from build123d import *

# Parameters (mm, degrees)
F0_W     = 3.2558272286
F0_H     = 15.3517797806
F1_DEPTH = 20
F2_R     = 2


with BuildPart() as f1:
    # F0 (on Top) → F1 (new body)
    with BuildSketch(Plane.XY):
        with BuildLine():
            Line((-40, -25), (40, -25))
            Line((40, -25), (40, 20))
            ThreePointArc((40, 20), (38.5355339059, 23.5355339059), (35, 25))
            Line((35, 25), (-35, 25))
            ThreePointArc((-35, 25), (-38.5355339059, 23.5355339059), (-40, 20))
            Line((-40, 20), (-40, -25))
        make_face()
        with BuildLine():
            Line((-12.7209101006, -4.8896298527), (-16.6285747722, -20.2414096333))
            Line((-16.6285747722, -20.2414096333), (-20.3346402347, -20.2414096333))
            Line((-20.3346402347, -20.2414096333), (-22.4144720763, -12.1774412653))
            add(Edge.make_bspline(
                [(-22.4144720763, -12.1774412653), (-22.5287116282, -11.7473629523), (-22.8075905342, -10.3983282441)],
                knots=[0, 0, 0, 1, 1, 1], degree=2))
            add(Edge.make_bspline(
                [(-22.8075905342, -10.3983282441), (-23.0864694403, -9.0492935358), (-23.1267892821, -8.5856153547)],
                knots=[0, 0, 0, 1, 1, 1], degree=2))
            add(Edge.make_bspline(
                [(-23.1267892821, -8.5856153547), (-23.1906290317, -9.1534531273), (-23.4426280432, -10.4084082045)],
                knots=[0, 0, 0, 1, 1, 1], degree=2))
            add(Edge.make_bspline(
                [(-23.4426280432, -10.4084082045), (-23.6946270547, -11.6633632818), (-23.8323865143, -12.1976011862)],
                knots=[0, 0, 0, 1, 1, 1], degree=2))
            Line((-23.8323865143, -12.1976011862), (-25.8987784087, -20.2414096333))
            Line((-25.8987784087, -20.2414096333), (-29.5947639107, -20.2414096333))
            Line((-29.5947639107, -20.2414096333), (-33.5125085428, -4.8896298527))
            Line((-33.5125085428, -4.8896298527), (-30.3104411033, -4.8896298527))
            Line((-30.3104411033, -4.8896298527), (-28.3448488136, -13.2694369818))
            add(Edge.make_bspline(
                [(-28.3448488136, -13.2694369818), (-27.8307708302, -15.5911878744), (-27.6022917264, -17.2913412053)],
                knots=[0, 0, 0, 1, 1, 1], degree=2))
            add(Edge.make_bspline(
                [(-27.6022917264, -17.2913412053), (-27.5384519768, -16.6932635514), (-27.3116528665, -15.4383084741)],
                knots=[0, 0, 0, 1, 1, 1], degree=2))
            add(Edge.make_bspline(
                [(-27.3116528665, -15.4383084741), (-27.0848537561, -14.1833533968), (-26.8866145337, -13.4911961119)],
                knots=[0, 0, 0, 1, 1, 1], degree=2))
            Line((-26.8866145337, -13.4911961119), (-24.6488633116, -4.8896298527))
            Line((-24.6488633116, -4.8896298527), (-21.5744753713, -4.8896298527))
            Line((-21.5744753713, -4.8896298527), (-19.3367241492, -13.4911961119))
            add(Edge.make_bspline(
                [(-19.3367241492, -13.4911961119), (-19.1888847291, -14.0657538581), (-18.9688055924, -15.253509199)],
                knots=[0, 0, 0, 1, 1, 1], degree=2))
            add(Edge.make_bspline(
                [(-18.9688055924, -15.253509199), (-18.7487264557, -16.4412645399), (-18.6344869038, -17.2913412053)],
                knots=[0, 0, 0, 1, 1, 1], degree=2))
            add(Edge.make_bspline(
                [(-18.6344869038, -17.2913412053), (-18.5303273124, -16.4715044213), (-18.2984882218, -15.2484692188)],
                knots=[0, 0, 0, 1, 1, 1], degree=2))
            add(Edge.make_bspline(
                [(-18.2984882218, -15.2484692188), (-18.0666491312, -14.0254340163), (-17.8784898693, -13.2694369818)],
                knots=[0, 0, 0, 1, 1, 1], degree=2))
            Line((-17.8784898693, -13.2694369818), (-15.9263375269, -4.8896298527))
            Line((-15.9263375269, -4.8896298527), (-12.7209101006, -4.8896298527))
        make_face(mode=Mode.SUBTRACT)
        with Locations((-9.1610040648, -12.565519743)):
            Rectangle(F0_W, F0_H, mode=Mode.SUBTRACT)
        Polygon((5.8127771986, -20.2414096333), (-3.6691056075, -20.2414096333), (-3.6691056075, -4.8896298527), (-0.4132783789, -4.8896298527), (-0.4132783789, -17.5534201773), (5.8127771986, -17.5534201773), align=None, mode=Mode.SUBTRACT)
        Polygon((17.9624895398, -20.2414096333), (8.4806067337, -20.2414096333), (8.4806067337, -4.8896298527), (11.7364339623, -4.8896298527), (11.7364339623, -17.5534201773), (17.9624895398, -17.5534201773), align=None, mode=Mode.SUBTRACT)
        Polygon((22.2263128144, -4.8896298527), (25.4082203329, -11.2097650611), (28.6102877724, -4.8896298527), (32.1181140125, -4.8896298527), (27.0243739934, -14.2673530673), (27.0243739934, -20.2414096333), (23.7920666725, -20.2414096333), (23.7920666725, -14.3715126587), (18.6983266534, -4.8896298527), align=None, mode=Mode.SUBTRACT)
    extrude(amount=F1_DEPTH)

    # F2
    f2_edges = [f1.edges().sort_by_distance(p)[0] for p in [
        (-40, -2.5, 20),
    ]]
    fillet(f2_edges, radius=F2_R)


solid = f1.part
Source: CAD feature listing. Evaluate the final solid. Frame: model axes, mm. Give positions to 0.01 mm unless a question says otherwise; leave off trailing zeros. Loops run counter-clockwise (first coordinate to the right, second up) from the corner with the lowest first, then second, coordinate; pieces in that order, holes last. Notation, with made-up numbers: (68.25, 40.5) -> (89.25, 40.5) arc R35 cw to (89.25, 75.5) -> close; hole circle Ø1 at (-7, 54.5). An arc over 180 degrees is marked (long way). Use a Markdown table: item, result. Add a question column.
1) Section query B-B, the plane y = -19. Count the separate pieces of the cut face and the enclosed holes in it, then the cut area to 3 significant figures.
2) Section query A-A, the plane x = 15.5. Return the cut outline in (y, z).
3) Line query: line 1 along Y through (x, z) = (3, 4.5); line 2 along Y through (x, z) = (30.5, 8); line 3 along X through (y, z) = (20.5, 6.5). Output: solid intervals per line, ascending. Write a range as [from, to].
4) Pull-direction query (Y, two-part tool) for faces 1 (the face through (-1, 0, 0)), 2 (the face through (25, -20.241, 10)), 3 (the face through (-10.789, -13, 10)); classes: +Y half, -Y half, draft (parallel to the pull), parting line (faces both ways), or undercut.
Numbers:
| question | item | result |
|---|---|---|
| 1 | separate pieces | 7 |
| 1 | enclosed holes | 0 |
| 1 | area | 916 mm2 |
| 2 | outline | (-25, 0) -> (-20.24, 0) -> (-20.24, 20) -> (-25, 20) -> close; (-17.55, 0) -> (25, 0) -> (25, 18) arc R2 ccw to (23, 20) -> (-17.55, 20) -> close |
| 3 | line 1 | y = [-25, -20.24], [-17.55, 25] |
| 3 | line 2 | y = [-25, -7.87], [-4.89, 25] |
| 3 | line 3 | x = [-39.97, 39.97] |
| 4 | face 1 | draft |
| 4 | face 2 | undercut |
| 4 | face 3 | undercut |
